Could you check a few things on this drawing? It's one solid part, dimensions in mm from its lowest x, y, z. A direction names the side the tool comes from. Give positions to 0.01 mm unless a question says otherwise; leave off trailing zeros. Order: outer loops, then holes, each group sorted by start corner. A loop starts at its lowest first (then second) coordinate and runs counter-clockwise, first axis right, second up. Notation, with made-up numbers: (31.25, 31.5) - (63.25, 31.5) arc R28 cw to (63.25, 50.5) - close; hole circle Ø10 at (35.25, -14). An arc over 180 degrees is marked (long way). Answer as CSV lines item,"result".
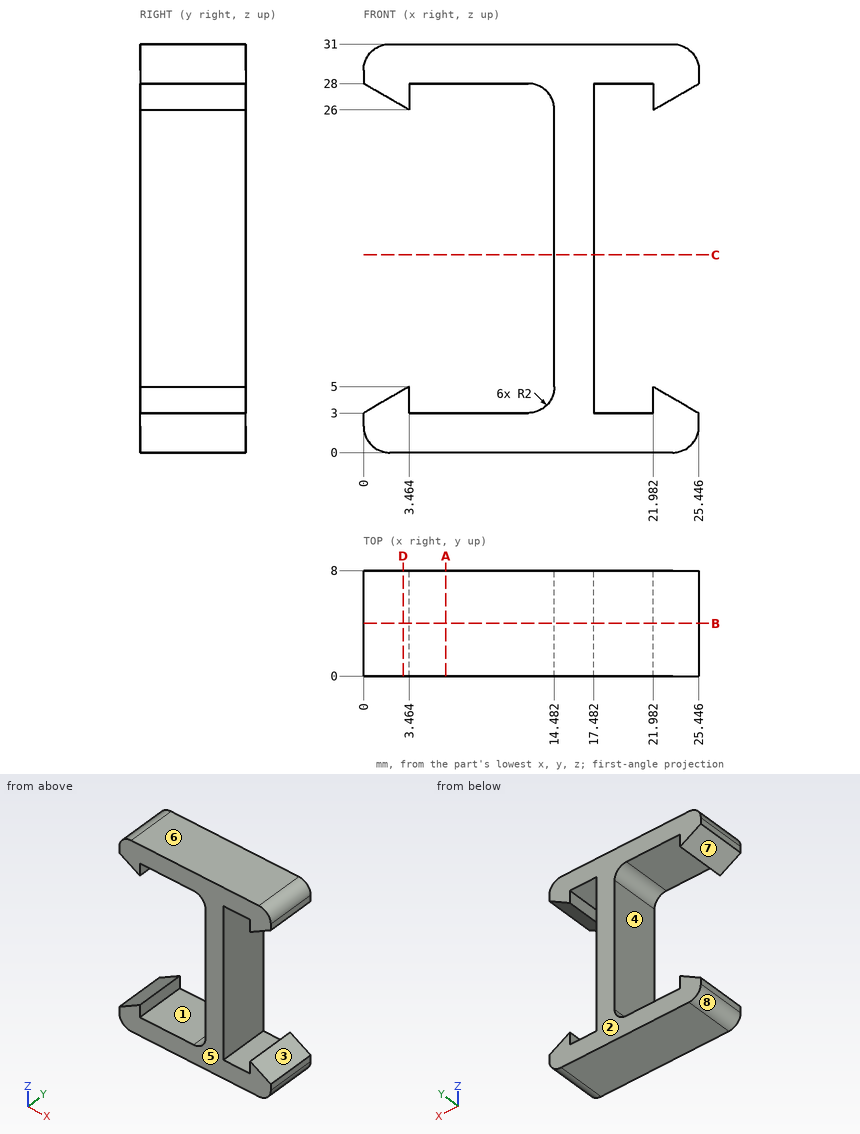
1) I want a section at C-C on z = 15. Write out the boundary of the cut face in (x, y).
Answer block:
outline,"(14.48, 0) - (17.48, 0) - (17.48, 8) - (14.48, 8) - close"
2) I want a section at D-D on x = 3. Write out the boundary of the cut face in (y, z).
Answer block:
outline,"(0, 0) - (8, 0) - (8, 4.73) - (0, 4.73) - close; (0, 26.27) - (8, 26.27) - (8, 31) - (0, 31) - close"
3) If we mould it in two halves opening along Z, with no side actions, what happens to the marked faces 6, 7 and 8? For each: +Z half, -Z half, draft (parallel to the pull), parting line (faces both ways), or undercut.
Answer block:
face 6,"+Z half"
face 7,"undercut"
face 8,"-Z half"
4) I want a section at A-A on x = 6.25. Write out the boundary of the cut face in (y, z), plus the area to 3 significant figures.
Answer block:
outline,"(0, 0) - (8, 0) - (8, 3) - (0, 3) - close; (0, 28) - (8, 28) - (8, 31) - (0, 31) - close"
area,"48.0 mm2"
5) I want a section at B-B on y = 4. Write out the boundary of the cut face in (x, z), plus the area to 3 significant figures.
Answer block:
outline,"(0, 2) arc R2 ccw to (2, 0) - (23.45, 0) arc R2 ccw to (25.45, 2) - (25.45, 3) - (21.98, 5) - (21.98, 3) - (17.48, 3) - (17.48, 28) - (21.98, 28) - (21.98, 26) - (25.45, 28) - (25.45, 29) arc R2 ccw to (23.45, 31) - (2, 31) arc R2 ccw to (0, 29) - (0, 28) - (3.46, 26) - (3.46, 28) - (12.48, 28) arc R2 cw to (14.48, 26) - (14.48, 5) arc R2 cw to (12.48, 3) - (3.46, 3) - (3.46, 5) - (0, 3) - close"
area,"240 mm2"
6) I'm going to push flat-ended pins straight in: P1, Ø4, axis at y = 3.5, z = 20, coming from the -X side; P2, Ø2, axis at y = 1, z = 4.5, coming from the -X side; P3, Ø0.6, axis at y = 3, z = 27, coming from the +X side. Where does each tip first touch, or does it pass through?
Answer block:
P1,"x = 14.48"
P2,"x = 0.87"
P3,"x = 24.23"
7) Which directions (+Z, -Z, +X, -X, +Y, -Y) give clear straight access to the entire face, cutting with the end or side of a thin tool? Please do the marked faces 1, 2, 3, 4 and 5.
Answer block:
face 1,"+Y, -Y"
face 2,"+Z, -Z, +X, -X, +Y"
face 3,"+X, +Y, -Y"
face 4,"-X, +Y, -Y"
face 5,"+Z, -Z, +X, -X, -Y"
8) I need wall thicknesses on line 1 along Z through (x, y) = (10.25, 6); line 2 along X through (y, z) = (6.25, 11); line 3 along Z through (x, y) = (22.75, 6.25). Which ranges of each line are inside material? Lowest first, please. Write a range as [from, to].
Answer block:
line 1,"[0, 3], [28, 31]"
line 2,"[14.48, 17.48]"
line 3,"[0, 4.56], [26.44, 31]"
